from build123d import *

# Parameters (mm, degrees)
SKETCH1_W           = 74.6
SKETCH1_H           = 86.6
BOSS_EXTRUDE1_DEPTH = 21
SHELL1_T            = -3
SKETCH3_R           = 2.9
SKETCH3_W           = 24.9
SKETCH3_H           = 20.6375
BOSS_EXTRUDE2_DEPTH = 3.175
FILLET2_R           = 4
BOSS_EXTRUDE3_DEPTH = 3
FILLET3_R           = 4
FILLET4_R           = 4
FILLET5_R           = 2
SKETCH5_W           = 12
SKETCH5_H           = 20
CUT_EXTRUDE1_DEPTH  = 37.3
CUT_EXTRUDE2_DEPTH  = 37.3
FILLET6_R           = 2
BOSS_EXTRUDE4_DEPTH = 21
FILLET7_R           = 2
FILLET8_R           = 2
SKETCH8_R           = 1.9
CUT_EXTRUDE3_DEPTH  = 5
SKETCH9_R           = 3.9
BOSS_EXTRUDE5_DEPTH = 21
FILLET9_R           = 1
CUT_EXTRUDE4_START  = -10
SKETCH10_R          = 1.9
CUT_EXTRUDE4_DEPTH  = 10


with BuildPart() as part:
    # Sketch1 → Boss-Extrude1 (new body)
    with BuildSketch(Plane(origin=(0, 0, 0), x_dir=(1, 0, 0), z_dir=(0, 1, 0))):
        Rectangle(SKETCH1_W, SKETCH1_H)
    extrude(amount=BOSS_EXTRUDE1_DEPTH)

    # Shell1
    shell1_openings = [part.faces().sort_by_distance(p)[0] for p in [
        (0, 21, 0),
    ]]
    offset(amount=SHELL1_T, openings=shell1_openings, kind=Kind.INTERSECTION)

    # Sketch3 → Boss-Extrude2 (add)
    with BuildSketch(Plane(origin=(0, 0, 0), x_dir=(1, 0, 0), z_dir=(0, 1, 0))):
        with BuildLine():
            Line((-37.3, -43.3), (-23.695893814, -72.433781099))
            ThreePointArc((-23.695893814, -72.433781099), (-21.518749084, -74.914349329), (-18.35, -75.8375))
            Line((-18.35, -75.8375), (18.35, -75.8375))
            ThreePointArc((18.35, -75.8375), (21.518749084, -74.914349329), (23.695893814, -72.433781099))
            Line((23.695893814, -72.433781099), (37.3, -43.3))
            Line((37.3, -43.3), (-37.3, -43.3))
        make_face()
        with Locations(Location((-18.35, -69.9375, 0), (0, 0, 270))):
            Circle(SKETCH3_R, mode=Mode.SUBTRACT)
        with Locations(Location((18.35, -69.9375, 0), (0, 0, 270))):
            Circle(SKETCH3_R, mode=Mode.SUBTRACT)
        with Locations(Location((18.35, -49.9375, 0), (0, 0, 270))):
            Circle(SKETCH3_R, mode=Mode.SUBTRACT)
        with Locations(Location((-18.35, -49.9375, 0), (0, 0, 270))):
            Circle(SKETCH3_R, mode=Mode.SUBTRACT)
        with Locations((0, -59.61875)):
            Rectangle(SKETCH3_W, SKETCH3_H, mode=Mode.SUBTRACT)
    extrude(amount=BOSS_EXTRUDE2_DEPTH)

    # Fillet2
    fillet2_edges = [part.edges().sort_by_distance(p)[0] for p in [
        (12.45, 1.5875, 69.9375),
        (12.45, 1.5875, 49.3),
        (-12.45, 1.5875, 49.3),
        (-12.45, 1.5875, 69.9375),
    ]]
    fillet(fillet2_edges, radius=FILLET2_R)

    # Sketch4 → Boss-Extrude3 (add)
    with BuildSketch(Plane(origin=(47.22244251, 0, 22.050660711), x_dir=(0.4230984913948713, 0, -0.9060836973367219), z_dir=(0.9060836973367219, 0, 0.4230984913948713))):
        Polygon((-23.451850366, 3.175), (-23.451850366, 21), (-48.451850366, 3.175), align=None)
    boss_extrude3 = extrude(amount=-BOSS_EXTRUDE3_DEPTH)

    # Mirror1: Boss-Extrude3 across plane
    add(boss_extrude3.mirror(Plane(origin=(0, 0, 0), x_dir=(0, 0, 1), z_dir=(1, 0, 0))))

    # Fillet3
    # the kernel refuses this fillet: 4 mm, written as the material it adds along each edge
    with BuildSketch(Plane(origin=(33.989047591, 35.70722548, 43.3), x_dir=(-1, 0, 0), z_dir=(0, -1, 0))) as fillet3_piece_1_section:
        with BuildLine():
            CenterArc((FILLET3_R * 1.57060379254, -FILLET3_R), FILLET3_R, 90, 115.030363343)
            Line((FILLET3_R * 0.664520095202, -FILLET3_R * 1.42309849139), (0, 0))
            Line((0, 0), (FILLET3_R * 1.57060379254, 0))
        make_face()
    fillet3_piece_1 = extrude(amount=32.53222548, mode=Mode.PRIVATE)
    fillet3_piece_1 = split(fillet3_piece_1, bisect_by=Plane(origin=(30.311758397, 15.920235221, 47.899774075), z_dir=(0.2456276241787504, -0.8142283147913327, -0.526022168384916)), keep=Keep.TOP, mode=Mode.PRIVATE)
    add(fillet3_piece_1)
    with BuildSketch(Plane(origin=(-33.989047591, 35.70722548, 43.3), x_dir=(1, 0, 0), z_dir=(0, -1, 0))) as fillet3_piece_2_section:
        with BuildLine():
            CenterArc((FILLET3_R * 1.57060379254, FILLET3_R), FILLET3_R, 154.969636657, 115.030363343)
            Line((FILLET3_R * 0.664520095202, FILLET3_R * 1.42309849139), (0, 0))
            Line((0, 0), (FILLET3_R * 1.57060379254, 0))
        make_face()
    fillet3_piece_2 = extrude(amount=32.53222548, mode=Mode.PRIVATE)
    fillet3_piece_2 = split(fillet3_piece_2, bisect_by=Plane(origin=(-30.311758397, 15.920235221, 47.899774075), z_dir=(-0.2456276241787504, -0.8142283147913327, -0.526022168384916)), keep=Keep.TOP, mode=Mode.PRIVATE)
    add(fillet3_piece_2)
    # the kernel refuses this fillet: 4 mm, written as the material it takes off along each edge
    with BuildSketch(Plane(origin=(37.3, -2.21972672, 43.3), x_dir=(0, 0, -1), z_dir=(0, 1, 0)), Plane(origin=(-37.3, -2.21972672, 43.3), x_dir=(0.42309849139487515, 0, 0.9060836973367199), z_dir=(0, 1, 0))) as fillet3_2_piece_1:
        with BuildLine():
            CenterArc((FILLET3_R * 0.221972672022, FILLET3_R), FILLET3_R, 244.969636657, 25.030363343)
            Line((-FILLET3_R * 0.201125819373, FILLET3_R * 0.0939163026633), (0, 0))
            Line((0, 0), (FILLET3_R * 0.221972672022, 0))
        make_face()
    extrude(amount=25.43945344, mode=Mode.SUBTRACT)
    with BuildSketch(Plane(origin=(-37.3, -10, -43.3), x_dir=(0, 0, 1), z_dir=(0, 1, 0))) as fillet3_2_piece_2:
        with BuildLine():
            CenterArc((FILLET3_R, FILLET3_R), FILLET3_R, 180, 90)
            Line((0, FILLET3_R), (0, 0))
            Line((0, 0), (FILLET3_R, 0))
        make_face()
    extrude(amount=41, mode=Mode.SUBTRACT)
    with BuildSketch(Plane(origin=(37.3, -10, -43.3), x_dir=(0, 0, 1), z_dir=(0, 1, 0))) as fillet3_2_piece_3:
        with BuildLine():
            CenterArc((FILLET3_R, -FILLET3_R), FILLET3_R, 90, 90)
            Line((0, -FILLET3_R), (0, 0))
            Line((0, 0), (FILLET3_R, 0))
        make_face()
    extrude(amount=41, mode=Mode.SUBTRACT)

    # Fillet4
    fillet4_edges = [part.edges().sort_by_distance(p)[0] for p in [
        (-25.363412169, 3.175, 65.317444696),
        (25.363412169, 3.175, 65.317444696),
    ]]
    fillet(fillet4_edges, radius=FILLET4_R)

    # Fillet5
    fillet5_edges = [part.edges().sort_by_distance(p)[0] for p in [
        (34.3, 12, 40.3),
        (34.3, 12, -40.3),
        (-34.3, 12, -40.3),
        (-34.3, 12, 40.3),
    ]]
    fillet(fillet5_edges, radius=FILLET5_R)

    # Sketch5 → Cut-Extrude1 (cut)
    with BuildSketch(Plane(origin=(0, 0, 0), x_dir=(0, 0, -1), z_dir=(1, 0, 0))):
        with Locations((26.5, 13)):
            Rectangle(SKETCH5_W, SKETCH5_H)
    extrude(amount=-CUT_EXTRUDE1_DEPTH, mode=Mode.SUBTRACT)

    # Sketch6 → Cut-Extrude2 (cut)
    with BuildSketch(Plane(origin=(0, 0, 0), x_dir=(0, 0, -1), z_dir=(1, 0, 0))):
        Polygon((29.5, 21), (17.5, 21), (17.5, 17), (17.5, 3), (29.5, 3), (29.5, 17), align=None)
    extrude(amount=CUT_EXTRUDE2_DEPTH, mode=Mode.SUBTRACT)

    # Fillet6
    fillet6_edges = [part.edges().sort_by_distance(p)[0] for p in [
        (-35.8, 21, -20.5),
        (-35.8, 21, -32.5),
        (-35.8, 3, -32.5),
        (-35.8, 3, -20.5),
        (35.8, 3, -29.5),
        (35.8, 3, -17.5),
        (35.8, 21, -17.5),
        (35.8, 21, -29.5),
    ]]
    fillet(fillet6_edges, radius=FILLET6_R)

    # Sketch7 → Boss-Extrude4 (add)
    with BuildSketch(Plane(origin=(0, 0, 0), x_dir=(1, 0, 0), z_dir=(0, 1, 0))):
        with BuildLine():
            Line((-37.3, 55.3), (-37.3, 39.3))
            ThreePointArc((-37.3, 39.3), (-36.128427125, 42.128427125), (-33.3, 43.3))
            Line((-33.3, 43.3), (-31.3, 43.3))
            Line((-31.3, 43.3), (-31.3, 55.3))
            Line((-31.3, 55.3), (-37.3, 55.3))
        make_face()
        with BuildLine():
            Line((31.3, 55.3), (31.3, 43.3))
            Line((31.3, 43.3), (33.3, 43.3))
            ThreePointArc((33.3, 43.3), (36.128427125, 42.128427125), (37.3, 39.3))
            Line((37.3, 39.3), (37.3, 55.3))
            Line((37.3, 55.3), (31.3, 55.3))
        make_face()
    extrude(amount=BOSS_EXTRUDE4_DEPTH)

    # Fillet7
    fillet7_edges = [part.edges().sort_by_distance(p)[0] for p in [
        (-37.3, 10.5, -55.3),
        (-31.3, 10.5, -55.3),
        (-31.3, 10.5, -43.3),
        (31.3, 10.5, -43.3),
        (31.3, 10.5, -55.3),
        (37.3, 10.5, -55.3),
    ]]
    fillet(fillet7_edges, radius=FILLET7_R)

    # Fillet8
    fillet8_edges = [part.edges().sort_by_distance(p)[0] for p in [
        (-27.396847741, 3.175, 57.417480766),
        (-31.08076756, 3.175, 45.151695536),
        (0, 3.175, 43.3),
        (31.08076756, 3.175, 45.151695536),
        (27.396847741, 3.175, 57.417480766),
    ]]
    fillet(fillet8_edges, radius=FILLET8_R)

    # Sketch8 → Cut-Extrude3 (cut)
    with BuildSketch(Plane(origin=(37.3, 0, 0), x_dir=(0, 0, -1), z_dir=(1, 0, 0))):
        with Locations((49.8, 5.096033911)):
            Circle(SKETCH8_R)
        with Locations((49.8, 17.096033911)):
            Circle(SKETCH8_R)
    cut_extrude3 = extrude(amount=-CUT_EXTRUDE3_DEPTH, mode=Mode.SUBTRACT)

    # Mirror2: Cut-Extrude3 across plane
    add(cut_extrude3.mirror(Plane(origin=(0, 0, 0), x_dir=(0, 0, 1), z_dir=(1, 0, 0))), mode=Mode.SUBTRACT)

    # Sketch9 → Boss-Extrude5 (add)
    with BuildSketch(Plane(origin=(0, 0, 0), x_dir=(1, 0, 0), z_dir=(0, 1, 0))):
        with Locations((33.4, 39.4)):
            Circle(SKETCH9_R)
        with Locations((-33.4, 39.4)):
            Circle(SKETCH9_R)
        with Locations((33.4, -39.4)):
            Circle(SKETCH9_R)
        with Locations((-33.4, -39.4)):
            Circle(SKETCH9_R)
    extrude(amount=BOSS_EXTRUDE5_DEPTH)

    # Fillet9
    fillet9_edges = [part.edges().sort_by_distance(p)[0] for p in [
        (34.3, 12, -35.605266808),
        (29.605266808, 12, -40.3),
        (-29.605266808, 12, -40.3),
        (-34.3, 12, -35.605266808),
        (29.605266808, 12, 40.3),
        (34.3, 12, 35.605266808),
        (-34.3, 12, 35.605266808),
        (-29.605266808, 12, 40.3),
    ]]
    fillet(fillet9_edges, radius=FILLET9_R)

    # Sketch10 → Cut-Extrude4 (cut)
    with BuildSketch(Plane(origin=(0, 21, 0), x_dir=(1, 0, 0), z_dir=(0, 1, 0)).offset(CUT_EXTRUDE4_START)):
        with Locations(Location((33.4, 39.4, 0), (0, 0, 270))):
            Circle(SKETCH10_R)
        with Locations(Location((-33.4, 39.4, 0), (0, 0, 270))):
            Circle(SKETCH10_R)
        with Locations(Location((-33.4, -39.4, 0), (0, 0, 270))):
            Circle(SKETCH10_R)
        with Locations(Location((33.4, -39.4, 0), (0, 0, 270))):
            Circle(SKETCH10_R)
    extrude(amount=CUT_EXTRUDE4_DEPTH, mode=Mode.SUBTRACT)


solid = part.part
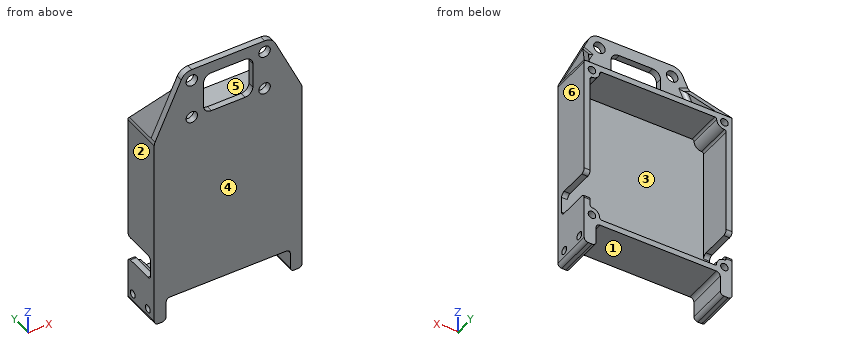
CAD build for the part. Positions are in the model's coordinates, mm. Face numbers are marked on the shaded views. A direction names the side the tool comes from. Give positions to 0.01 mm unless a question says otherwise; leave off trailing zeros. Order: outer loops, then holes, each group sorted by start corner. A loop starts at its lowest first (then second) coordinate and runs counter-clockwise, first axis right, second up. Notation, with made-up numbers: (-25.75, -40) - (20.25, -40) arc R17 cw to (20.25, -11) - close; hole circle Ø4 at (17, -5). An arc over 180 degrees is marked (long way). Answer in a Markdown table with one row per item.
1. Saw through at B-B, the plane x = -6. Give the cut face in (y, z) (1 decimal), plus the area to 3 significant figures.
Data:
| item | result |
|---|---|
| outline | (0, -43.3) - (21, -43.3) - (21, -40.3) - (3, -40.3) - (3, 40.3) - (21, 40.3) - (21, 43.3) - (5.2, 43.3) arc R2 cw to (3.2, 45.3) - (3.2, 49.3) - (0, 49.3) - close; (0, 69.9) - (3.2, 69.9) - (3.2, 75.8) - (0, 75.8) - close |
| area | 406 mm² |
2. Probe probe 1 along Y at (x, z) = (-35.25, -49.8); probe 2 along X at (y, z) = (15.5, 39.4); probe 3 along Z at (x, y) = (-26, 17.75). List the from-to ranges inside material, lowest first. Write a range as [from, to].
Data:
| item | result |
|---|---|
| probe 1 | y = [0, 3.2], [7, 15.2], [19, 21] |
| probe 2 | x = [-37.3, -35.3], [-31.5, -29.5], [29.5, 31.5], [35.3, 37.3] |
| probe 3 | z = [-43.3, -40.3], [40.3, 43.3] |
3. Saw through at D-D, the plane z = -24. Give the cut face in (x, y), plus the area to 3 significant figures.
Data:
| item | result |
|---|---|
| outline | (-37.3, 0) - (37.3, 0) - (37.3, 3) - (-37.3, 3) - close |
| area | 224 mm² |
4. Saw through at A-A, the plane z = -49.8. Give the cut face in (x, y).
Data:
| item | result |
|---|---|
| outline | (-37.3, 0) - (-31.3, 0) - (-31.3, 21) - (-37.3, 21) - (-37.3, 19) - (-32.3, 19) - (-32.3, 15.2) - (-37.3, 15.2) - (-37.3, 7) - (-32.3, 7) - (-32.3, 3.2) - (-37.3, 3.2) - close; (31.3, 0) - (37.3, 0) - (37.3, 3.2) - (32.3, 3.2) - (32.3, 7) - (37.3, 7) - (37.3, 15.2) - (32.3, 15.2) - (32.3, 19) - (37.3, 19) - (37.3, 21) - (31.3, 21) - close |
5. Saw through at C-C, the plane x = 17. Give the cut face in (y, z) (1 decimal).
Data:
| item | result |
|---|---|
| outline | (0, -43.3) - (21, -43.3) - (21, -40.3) - (3, -40.3) - (3, 40.3) - (21, 40.3) - (21, 43.3) - (5.2, 43.3) arc R2 cw to (3.2, 45.3) - (3.2, 47.4) - (0, 47.4) - close; (0, 52.5) - (3.2, 52.5) - (3.2, 67.4) - (0, 67.4) - close; (0, 72.5) - (3.2, 72.5) - (3.2, 75.8) - (0, 75.8) - close |
6. Flat gauge pins, fed straight in: pin 1 (2 mm diameter, centred on x = -8, z = -23.5, fed in from +Y); pin 2 (3 mm diameter, centred on y = 5.1, z = -49.8, fed in from -X); pin 3 (5 mm diameter, centred on x = -18.35, z = 69.94, fed in from -Y); pin 4 (10 mm diameter, centred on x = 12, y = 18.5, fed in from -Z). Where does each tip first touch, or does it go through?
Data:
| item | result |
|---|---|
| pin 1 | stops at y = 3 |
| pin 2 | stops at x = -32.3 |
| pin 3 | passes through |
| pin 4 | stops at z = -43.3 |
7. Pull direction X, two halves, no side cores. Call the marked faces 4, 5 and 6: pulls with the +X half, pulls with the -X half, needs draft (parallel to the pull), parting line crosses it, or undercut.
Data:
| item | result |
|---|---|
| face 4 | needs draft |
| face 5 | undercut |
| face 6 | pulls with the +X half |
8. Tool access for the marked faces 1, 2 and 3: list every direction of +Z, -Z, +X, -X, +Y, -Y with a clear straight run to the whole face (end or side of a thin tool).
Data:
| item | result |
|---|---|
| face 1 | -Z, +Y, -Y |
| face 2 | +Z, -Z, -X, +Y, -Y |
| face 3 | +Y |
